Could you check a few things on this model? Use its own coordinates, in mm. Face numbers are marked on the shaded views. A direction names the side the tool comes from. Give positions to 0.01 mm unless a question says otherwise; leave off trailing zeros. Write each loop counter-clockwise with the first axis right and the second up, starting at its lowest first coordinate (ties: lowest second). Pieces come first, ordered by that corner, then holes. Notation, with made-up numbers: M 39.5,25.25 L 45.5,25.25 A20 ccw 45.5,30.25 Z; hole C 60.25,27 d1. An arc over 180 degrees is marked long. Write each question's results on one line, items separated by ' | '. Start each with the question number.
from build123d import *

# Parameters (mm, degrees)
EXTRUDE_1_DEPTH          = 8
SKETCH_3_W               = 42
SKETCH_3_H               = 3
EXTRUDE_2_DEPTH          = 43
CUT_EXTRUDE_1_REACH      = 78
SKETCH_4_R               = 1.5
SKETCH_5_W               = 25
SKETCH_5_H               = 17
CUT_EXTRUDE_2_DEPTH      = 9
SKETCH_7_R               = 3
CUT_EXTRUDE_3_DEPTH      = 9
FILLET_1_R               = 5
CUT_EXTRUDE_4_DEPTH      = 9
SKETCH_9_R               = 1.5
CUT_EXTRUDE_5_DEPTH      = 1
CUT_EXTRUDE_5_DEPTH_BACK = 81
SKETCH_12_W              = 80
SKETCH_12_H              = 25
EXTRUDE_4_DEPTH          = 45
SKETCH_13_W              = 6
SKETCH_13_H              = 25
CUT_EXTRUDE_6_DEPTH      = 42
FILLET_3_R               = 5
FILLET_4_R               = 5


with BuildPart() as part:
    # 草图1 → 凸台-拉伸1 (new body)
    with BuildSketch(Plane.XY):
        Polygon((-40, -42.5), (40, -42.5), (40, 42.5), (40, 50.5), (-40, 50.5), (-40, 42.5), align=None)
    extrude(amount=EXTRUDE_1_DEPTH)

    # 草图3 → 凸台-拉伸2 (add)
    with BuildSketch(Plane.XY.offset(8)):
        with Locations((0, -24)):
            Rectangle(SKETCH_3_W, SKETCH_3_H)
    extrude(amount=EXTRUDE_2_DEPTH)

    # 草图4 → 切除-拉伸1 (cut, up to next)
    with BuildSketch(Plane.XZ.offset(25.5), mode=Mode.PRIVATE) as cut_extrude_1_sk1:
        with Locations((-15.5, 44.5)):
            Circle(SKETCH_4_R)
    cut_extrude_1_tool1 = extrude(cut_extrude_1_sk1.sketch, amount=-CUT_EXTRUDE_1_REACH, mode=Mode.PRIVATE) & part.part
    add(cut_extrude_1_tool1.solids().sort_by_distance((-15.5, -25.5, 44.5))[0], mode=Mode.SUBTRACT)
    # 草图4 → 切除-拉伸1 (cut, up to next)
    with BuildSketch(Plane.XZ.offset(25.5), mode=Mode.PRIVATE) as cut_extrude_1_sk2:
        with Locations((15.5, 44.5)):
            Circle(SKETCH_4_R)
    cut_extrude_1_tool2 = extrude(cut_extrude_1_sk2.sketch, amount=-CUT_EXTRUDE_1_REACH, mode=Mode.PRIVATE) & part.part
    add(cut_extrude_1_tool2.solids().sort_by_distance((15.5, -25.5, 44.5))[0], mode=Mode.SUBTRACT)
    # 草图4 → 切除-拉伸1 (cut, up to next)
    with BuildSketch(Plane.XZ.offset(25.5), mode=Mode.PRIVATE) as cut_extrude_1_sk3:
        with Locations((15.5, 13.5)):
            Circle(SKETCH_4_R)
    cut_extrude_1_tool3 = extrude(cut_extrude_1_sk3.sketch, amount=-CUT_EXTRUDE_1_REACH, mode=Mode.PRIVATE) & part.part
    add(cut_extrude_1_tool3.solids().sort_by_distance((15.5, -25.5, 13.5))[0], mode=Mode.SUBTRACT)
    # 草图4 → 切除-拉伸1 (cut, up to next)
    with BuildSketch(Plane.XZ.offset(25.5), mode=Mode.PRIVATE) as cut_extrude_1_sk4:
        with Locations((-15.5, 13.5)):
            Circle(SKETCH_4_R)
    cut_extrude_1_tool4 = extrude(cut_extrude_1_sk4.sketch, amount=-CUT_EXTRUDE_1_REACH, mode=Mode.PRIVATE) & part.part
    add(cut_extrude_1_tool4.solids().sort_by_distance((-15.5, -25.5, 13.5))[0], mode=Mode.SUBTRACT)
    # 草图4 → 切除-拉伸1 (cut, up to next)
    with BuildSketch(Plane.XZ.offset(25.5), mode=Mode.PRIVATE) as cut_extrude_1_sk5:
        with BuildLine():
            Line((-11, 29), (-11, 51))
            Line((-11, 51), (11, 51))
            Line((11, 51), (11, 29))
            ThreePointArc((11, 29), (0, 18), (-11, 29))
        make_face()
    cut_extrude_1_tool5 = extrude(cut_extrude_1_sk5.sketch, amount=-CUT_EXTRUDE_1_REACH, mode=Mode.PRIVATE) & part.part
    add(cut_extrude_1_tool5.solids().sort_by_distance((0, -25.5, 35.581943))[0], mode=Mode.SUBTRACT)

    # 草图5 → 切除-拉伸2 (cut, through all)
    with BuildSketch(Plane.XY.offset(8)):
        with Locations((0, -34)):
            Rectangle(SKETCH_5_W, SKETCH_5_H)
    extrude(amount=-CUT_EXTRUDE_2_DEPTH, mode=Mode.SUBTRACT)

    # 草图7 → 切除-拉伸3 (cut, through all)
    with BuildSketch(Plane.XY.offset(8)):
        with Locations((-25, 17.5)):
            Circle(SKETCH_7_R)
        with Locations((25, 17.5)):
            Circle(SKETCH_7_R)
        with Locations((-25, -22.25)):
            Circle(SKETCH_7_R)
        with Locations((25, -22.25)):
            Circle(SKETCH_7_R)
    extrude(amount=-CUT_EXTRUDE_3_DEPTH, mode=Mode.SUBTRACT)

    # 圆角1
    fillet_1_edges = [part.edges().sort_by_distance(p)[0] for p in [
        (-40, -42.5, 4),
    ]]
    fillet(fillet_1_edges, radius=FILLET_1_R)

    # 草图8 → 切除-拉伸4 (cut, through all)
    with BuildSketch(Plane.XY.offset(8)):
        with BuildLine():
            Line((-28, -22.25), (-28, -42.5))
            Line((-28, -42.5), (-27, -42.5))
            Line((-27, -42.5), (-27, -24.486067977))
            ThreePointArc((-27, -24.486067977), (-27.738612788, -23.474744871), (-28, -22.25))
        make_face()
        with BuildLine():
            Line((28, -42.5), (27, -42.5))
            Line((27, -42.5), (27, -24.486067977))
            ThreePointArc((27, -24.486067977), (27.738612788, -23.474744871), (28, -22.25))
            Line((28, -22.25), (28, -42.5))
        make_face()
    extrude(amount=-CUT_EXTRUDE_4_DEPTH, mode=Mode.SUBTRACT)

    # 草图9 → 切除-拉伸5 (cut, two sides)
    with BuildSketch(Plane.ZY.offset(40)) as cut_extrude_5_sk:
        with Locations((4, -35.5)):
            Circle(SKETCH_9_R)
    extrude(amount=CUT_EXTRUDE_5_DEPTH, mode=Mode.SUBTRACT)
    extrude(cut_extrude_5_sk.sketch, amount=-CUT_EXTRUDE_5_DEPTH_BACK, mode=Mode.SUBTRACT)

    # 草图12 → 凸台-拉伸4 (add)
    with BuildSketch(Plane.XY.offset(8)):
        with Locations((0, 38)):
            Rectangle(SKETCH_12_W, SKETCH_12_H)
    extrude(amount=EXTRUDE_4_DEPTH)

    # 草图13 → 切除-拉伸6 (cut)
    with BuildSketch(Plane.XY.offset(53)):
        with Locations((0, 38)):
            Rectangle(SKETCH_13_W, SKETCH_13_H)
    extrude(amount=-CUT_EXTRUDE_6_DEPTH, mode=Mode.SUBTRACT)

    # 圆角3
    fillet_3_edges = [part.edges().sort_by_distance(p)[0] for p in [
        (-40, 25.5, 30.5),
        (40, 25.5, 30.5),
    ]]
    fillet(fillet_3_edges, radius=FILLET_3_R)

    # 圆角4
    fillet_4_edges = [part.edges().sort_by_distance(p)[0] for p in [
        (40, -42.5, 4),
    ]]
    fillet(fillet_4_edges, radius=FILLET_4_R)


solid = part.part
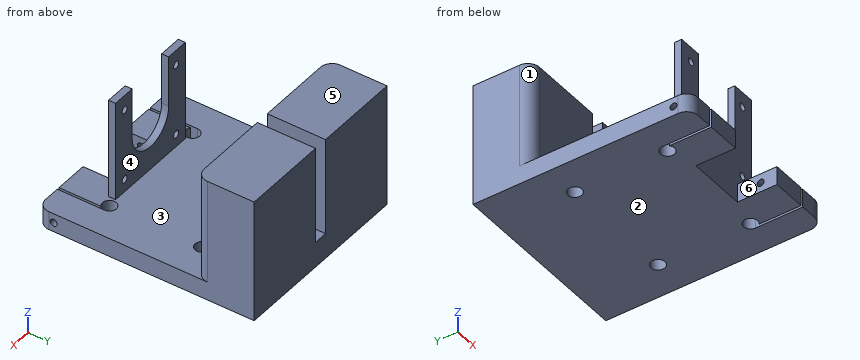
Q1. For the marked faces 4, 5 and 6, which set-ups out of +Z, -Z, +X, -X, +Y, -Y let a thin tool reach every point of the face, with its end or its side?
Q2. I'm going to push flat-ended pins straight in: P1, Ø3.5, axis at x = 13.5, y = -23.5, coming from the +Z side; P2, Ø10, axis at x = 14.5, y = 4, coming from the +Z side; P3, Ø2.5, axis at x = 15.5, z = 13.5, coming from the -Y side. Where does each tip first touch, or does it pass through?
Q3. If we section it at C-C (z = 44.5): Please give me the cut outline in (x, y), plus the area to 3 significant figures.
Q4. Please list where these lines run through material, in increasing order: line 1 (Z direction, x = -15.5, y = -24.3); line 2 (Y direction, x = 25, z = 3.5); line 3 (Y direction, x = -10, z = 14). Write a range as [from, to].
Q5. If we mould it in two halves opening along Y, with no side actions, what happens to the marked faces 1, 2 and 3? For each: pulls with the +Y half, pulls with the -Y half, needs draft (parallel to the pull), parting line crosses it, or undercut.
Q6. If we section it at B-B (y = 17.5): Please give me the cut outline in (x, z).
Q7. If we section it at A-A (x = 15.5): Please give me the cut outline in (y, z), plus the area to 3 significant figures.
Q8. If we section it at D-D (y = -35.5): Count the separate pieces of the cut face and the enclosed holes in it, plus the area to 3 significant figures.
Determined:
1) face 4: +Z, +X, -X | face 5: +Z, +X, -X, +Y, -Y | face 6: +Z, -Z, -Y
2) P1: stops at z = 51 | P2: stops at z = 8 | P3: stops at y = 25.5
3) outline: M -40,30.5 A5 ccw -35,25.5 L -3,25.5 L -3,50.5 L -40,50.5 Z; M -21,-25.5 L -17,-25.5 L -17,-22.5 L -21,-22.5 Z; M -14,-25.5 L -11,-25.5 L -11,-22.5 L -14,-22.5 Z; M 3,25.5 L 35,25.5 A5 ccw 40,30.5 L 40,50.5 L 3,50.5 Z; M 11,-25.5 L 14,-25.5 L 14,-22.5 L 11,-22.5 Z; M 17,-25.5 L 21,-25.5 L 21,-22.5 L 17,-22.5 Z | area: 1,880 mm²
4) line 1: z = [0, 12], [15, 43], [46, 51] | line 2: y = [-42.5, -36.91], [-34.09, -25.25], [-19.25, 14.5], [20.5, 50.5] | line 3: y = [-25.5, -22.5], [25.5, 50.5]
5) face 1: pulls with the -Y half | face 2: needs draft | face 3: undercut
6) outline: M -40,0 L -28,0 L -28,8 L -40,8 Z; M -22,0 L 22,0 L 22,8 L -22,8 Z; M 28,0 L 40,0 L 40,8 L 28,8 Z
7) outline: M -42.5,0 L 50.5,0 L 50.5,53 L 25.5,53 L 25.5,8 L -22.5,8 L -22.5,12 L -25.5,12 L -25.5,8 L -42.5,8 Z; M -25.5,15 L -22.5,15 L -22.5,43 L -25.5,43 Z; M -25.5,46 L -22.5,46 L -22.5,51 L -25.5,51 Z; hole C -35.5,4 d3 | area: 1,970 mm²
8) separate pieces: 8 | enclosed holes: 0 | area: 265 mm²
